```python
from build123d import *

# Parameters (mm, degrees)
SKETCH2_R           = 116.84
BOSS_EXTRUDE1_DEPTH = 1.5875


with BuildPart() as part:
    # Sketch2 → Boss-Extrude1 (new, symmetric)
    with BuildSketch(Plane.XY):
        with BuildLine():
            ThreePointArc((-1.651, 128.513680847), (-113.44208216, 64.09028885), (-116.977106193, -64.886930424))
            ThreePointArc((-116.977106193, -64.886930424), (-116.59127356, -65.61727077), (-116.200881143, -66.345183954))
            ThreePointArc((-116.200881143, -66.345183954), (-115.806084025, -67.070386581), (-115.406761019, -67.793106963))
            ThreePointArc((-115.406761019, -67.793106963), (0, -135.636), (115.406761019, -67.793106963))
            ThreePointArc((115.406761019, -67.793106963), (115.804512811, -67.073251299), (116.197774523, -66.350932884))
            ThreePointArc((116.197774523, -66.350932884), (116.589738292, -65.620154913), (116.977106193, -64.886930424))
            ThreePointArc((116.977106193, -64.886930424), (113.44208216, 64.09028885), (1.651, 128.513680847))
            ThreePointArc((1.651, 128.513680847), (0.825516124, 128.521420187), (0, 128.524))
            ThreePointArc((0, 128.524), (-0.825516124, 128.521420187), (-1.651, 128.513680847))
        make_face()
        with Locations((0, -3.556)):
            Circle(SKETCH2_R, mode=Mode.SUBTRACT)
    extrude(amount=BOSS_EXTRUDE1_DEPTH, both=True)


solid = part.part
```
Part model, mm, in its own coordinate system. Give positions to 0.01 mm unless a question says otherwise; leave off trailing zeros. Write each loop counter-clockwise with the first axis right and the second up, starting at its lowest first coordinate (ties: lowest second). Pieces come first, ordered by that corner, then holes. Notation, with made-up numbers: (12, -25.75) -> (33, -25.75) arc R24 cw to (33, 0.25) -> close; hole circle Ø11 at (15, -11). An arc over 180 degrees is marked (long way). Put each result on its own line as item: value. Start each with the question number.
Item 1: Pull direction X, two halves, no side cores. Call faces 1 (the face through (-112.464, 65.704, 0.022)), 2 (the face through (-86.116, 75.41, -0.022)), 3 (the face through (9.2, -120.3, 1.588)): pulls with the +X half, pulls with the -X half, needs draft (parallel to the pull), parting line crosses it, or undercut.
Item 2: Pin check, flat tips, straight feed: pin 1 Ø1.5 at (y, z) = (-70.5, 0.5) entering from -X; pin 2 Ø1 at (y, z) = (5, 1) entering from +X; pin 3 Ø1 at (x, z) = (-103.5, 0.5) entering from +Y. Stop position of each tip, or through.
Item 3: Cut at A-A (y = 107). List the corners of the cut face in (x, z).
Item 4: Cut at C-C (z = 0.15). List the corners of the cut face in (x, y).
Item 5: Cut at B-B (x = -36). List the corners of the cut face in (y, z), then the cut area to 3 significant figures.
Item 6: Wall check: L1, parallel to Y at x = 0, z = 0.6; L2, parallel to X at y = -17.5, z = 0.9; L3, parallel to X at y = 18, z = 0.2. Give the ranges that are in metal, low to high. Write a range as [from, to].
Answer list:
1. face 1: pulls with the -X half
1. face 2: undercut
1. face 3: needs draft
2. pin 1: stops at x = -114.3
2. pin 2: stops at x = 131.83
2. pin 3: stops at y = 79.12
3. outline: (-72.27, -1.59) -> (-37.8, -1.59) -> (-37.8, 1.59) -> (-72.27, 1.59) -> close; (37.8, -1.59) -> (72.27, -1.59) -> (72.27, 1.59) -> (37.8, 1.59) -> close
4. outline: (-116.98, -64.89) arc R132.08 ccw to (-116.2, -66.35) arc R132.08 ccw to (-115.41, -67.79) arc R132.08 ccw to (115.41, -67.79) arc R132.08 ccw to (116.2, -66.35) arc R132.08 ccw to (116.98, -64.89) arc R132.08 ccw to (1.65, 128.51) arc R132.08 ccw to (-1.65, 128.51) arc R132.08 ccw to start; hole circle Ø233.68 at (0, -3.56)
5. outline: (-130.64, -1.59) -> (-114.71, -1.59) -> (-114.71, 1.59) -> (-130.64, 1.59) -> close; (107.6, -1.59) -> (123.52, -1.59) -> (123.52, 1.59) -> (107.6, 1.59) -> close
5. area: 101 mm2
6. L1: y = [-135.64, -120.4], [113.28, 128.52]
6. L2: x = [-131.34, -116], [116, 131.34]
6. L3: x = [-130.31, -114.83], [114.83, 130.31]
